from build123d import *

# Parameters (mm, degrees)
SKETCH1_W           = 30
SKETCH1_H           = 30
BOSS_EXTRUDE1_DEPTH = 3
SKETCH2_W           = 5
SKETCH2_H           = 3
SKETCH2_W_2         = 1.313790547
SKETCH2_W_3         = 3
SKETCH2_H_2         = 4
CUT_EXTRUDE1_DEPTH  = 3
SKETCH3_W           = 3.847981768
SKETCH3_H           = 13.294575909
CUT_EXTRUDE2_DEPTH  = 3
CUT_EXTRUDE3_DEPTH  = 3
CUT_EXTRUDE4_DEPTH  = 10


with BuildPart() as part:
    # Sketch1 → Boss-Extrude1 (new body)
    with BuildSketch(Plane(origin=(0, 0, 0), x_dir=(1, 0, 0), z_dir=(0, 1, 0))):
        with Locations((15, -15)):
            Rectangle(SKETCH1_W, SKETCH1_H)
    extrude(amount=BOSS_EXTRUDE1_DEPTH)

    # Sketch2 → Cut-Extrude1 (cut)
    with BuildSketch(Plane.XZ):
        with Locations((10.5, 1.5)):
            Rectangle(SKETCH2_W, SKETCH2_H)
        with Locations((25.043104727, 1.5)):
            Rectangle(SKETCH2_W_2, SKETCH2_H)
        with Locations((1.5, 1.5)):
            Rectangle(SKETCH2_W_3, SKETCH2_H)
        with Locations((1.5, 8)):
            Rectangle(SKETCH2_W_3, SKETCH2_H_2)
    extrude(amount=-CUT_EXTRUDE1_DEPTH, mode=Mode.SUBTRACT)

    # Sketch3 → Cut-Extrude2 (cut)
    with BuildSketch(Plane.XZ):
        with Locations((20.035652011, 9.340199914)):
            Rectangle(SKETCH3_W, SKETCH3_H)
    extrude(amount=-CUT_EXTRUDE2_DEPTH, mode=Mode.SUBTRACT)

    # Sketch4 → Cut-Extrude3 (cut)
    with BuildSketch(Plane.XZ):
        Polygon((0, 14.83898954), (4.273286448, 14.83898954), (4.273286448, 17.83898954), (7.572046642, 17.83898954), (7.572046642, 14.83898954), (12.983097177, 14.83898954), (12.983097177, 17.83898954), (18.173549861, 17.83898954), (18.111661127, 14.83898954), (30, 15), (30, 36.64216365), (-3.662569557, 36.64216365), (-3.662569557, 14.83898954), align=None)
    extrude(amount=-CUT_EXTRUDE3_DEPTH, mode=Mode.SUBTRACT)

    # Sketch6 → Cut-Extrude4 (cut)
    with BuildSketch(Plane(origin=(0, 3, 0), x_dir=(1, 0, 0), z_dir=(0, 1, 0))):
        Polygon((25.7, 0), (25.7, -20.065163227), (34.530029549, -19.489635477), (33.156944601, 1.576908509), (28.640882237, 2.839466423), align=None)
    extrude(amount=-CUT_EXTRUDE4_DEPTH, mode=Mode.SUBTRACT)


solid = part.part
Source: CAD feature listing. Evaluate the final solid. Frame: model axes, mm. A direction names the side the tool comes from. Coordinates: 2 decimals unless noted, no trailing zeros. Order: outer loops, then holes, each group sorted by start corner. A loop starts at its lowest first (then second) coordinate and runs counter-clockwise, first axis right, second up. Notation, with made-up numbers: M 31.5,-35 L 44.5,-35 A20 cw 44.5,-11 Z; hole C 18.25,70.5 d6. An arc over 180 degrees is marked long. Write each question's results on one line, items separated by ' | '. Start each with the question number.
Item 1: Draft query along Z for faces 4 (the face through (25.7, 2, 9)), 5 (the face through (18.112, 1, 9)), 6 (the face through (5, 1, 0)). Return one class per face: pulls with the +Z half, pulls with the -Z half, needs draft (parallel to the pull), parting line crosses it, or undercut.
Item 2: Cut plane A-A (z = 15.5). Return loops of the section in (x, y).
Item 3: Cut plane B-B (x = 2.5). Return loops of the section in (y, z).
Item 4: Line query: probe 1 along X at (y, z) = (1.8, 13.25); probe 2 along Z at (x, y) = (2.75, 0.8); probe 3 along X at (y, z) = (1.45, 2.75). Output: solid intervals per line, ascending.
Item 5: Cut plane D-D (x = 19.25). Return loops of the section in (y, z).
Item 6: First-contact query: pin 1 Ø0.9 at (y, z) = (1, 1.5) entering from +X; pin 2 Ø0.9 at (y, z) = (1.5, 9.5) entering from -X; pin 3 Ø1.5 at (y, z) = (1.5, 17) entering from -X. Flat tips, straight axial feed; report the tip coordinate or a pass-through.
Item 7: Set-up query: faces 1 (the face through (25, 1, 3)), 2 (the face through (1, 1, 3)), 3 (the face through (2, 1, 14.839)). Return all of +Z, -Z, +X, -X, +Y, -Y with unobstructed straight access to the full face (end or side cutting, diameter ignored); none if empty.
Checked values:
1) face 4: needs draft | face 5: undercut | face 6: pulls with the -Z half
2) outline: M 4.27,0 L 7.57,0 L 7.57,3 L 4.27,3 Z; M 12.98,0 L 18.11,0 L 18.11,3 L 12.98,3 Z
3) outline: M 0,3 L 3,3 L 3,6 L 0,6 Z; M 0,10 L 3,10 L 3,14.84 L 0,14.84 Z
4) probe 1: x = 0 to 18.11, 21.96 to 25.7 | probe 2: z = 3 to 6, 10 to 14.84 | probe 3: x = 3 to 8, 13 to 18.11, 21.96 to 24.39
5) outline: M 0,0 L 3,0 L 3,2.69 L 0,2.69 Z
6) pin 1: stops at x = 24.39 | pin 2: stops at x = 3 | pin 3: stops at x = 4.27
7) face 1: -Z, +X, +Y, -Y | face 2: -Z, -X, +Y, -Y | face 3: +Z, -X, +Y, -Y
